```python
from build123d import *

# Parameters (mm, degrees)
F0_R      = 2
F0_R_2    = 1.25
F1_DEPTH  = 2.5
F2_DEPTH  = 8.5
F3_R      = 1.25
F2_FACE_R = 1.25
F4_DEPTH  = 1.5
F5_R      = 0.25


with BuildPart() as f1:
    # F0 (on Top) → F1 (new body)
    with BuildSketch(Plane.XY):
        Circle(F0_R)
        Circle(F0_R_2, mode=Mode.SUBTRACT)
    extrude(amount=F1_DEPTH)

    # F0 (on Top) → F2 (join)
    with BuildSketch(Plane.XY):
        Circle(F0_R_2)
    extrude(amount=F2_DEPTH)

    # F0 (on Top) + F3 (on face) + F2_face (on face) → F4 (cut)
    with BuildSketch(Plane.XY):
        Circle(F0_R_2)
    with BuildSketch(Plane.XY):
        Polygon((-0.8660254038, -1.5), (0.8660254038, -1.5), (1.7320508076, 0), (0.8660254038, 1.5), (-0.8660254038, 1.5), (-1.7320508076, 0), align=None)
        Circle(F3_R, mode=Mode.SUBTRACT)
        Circle(F3_R)
    with BuildSketch(Plane.XY.offset(8.5)):
        Circle(F2_FACE_R)
    extrude(amount=F4_DEPTH, mode=Mode.SUBTRACT)

    # F5
    f5_edges = [f1.edges().sort_by_distance(p)[0] for p in [
        (-1.25, 0, 2.5),
        (-2, 0, 2.5),
        (-2, 0, 0),
    ]]
    fillet(f5_edges, radius=F5_R)


solid = f1.part
```
Verification items for the finished model (mm, model axes). A direction names the side the tool comes from. Round coordinates to 2 decimals unless told otherwise and drop trailing zeros. Write each loop counter-clockwise with the first axis right and the second up, starting at its lowest first coordinate (ties: lowest second). Pieces come first, ordered by that corner, then holes.
1. Gauge pin test, flat ends, axial feed: P1, Ø2, axis at x = -1, z = 5, coming from the -Y side; P2, Ø1.5, axis at x = -0.5, y = 0.5, coming from the -Z side. Record the tip position at first contact, or that the pin passes through.
2. Scan lines: L1, parallel to X at y = -0.9, z = 1; L2, parallel to Z at x = 1.45, y = -0.9; L3, parallel to Z at x = 0.15, y = 0.95. Record each from-to range of solid material in increasing order.
3. Access from +Z, -Z, +X, -X, +Y, -Y to the whole of each face (thin tool, end or side, straight path). Record for faces 4 (the flat face through (0, -1.5, 1)), 5 (the cylindrical face through (0, -2, 1)).
4. Draft check along X on faces 1 (the flat face through (-1.305, -0.74, 0.74)), 2 (the cylindrical face through (-0.27, -1.22, 5.58)), 3 (the flat face through (0, 0, 8.5)). Enter one of: +X half, -X half, draft (parallel to the pull), parting line (faces both ways), or undercut.
5. Section check A-A on x = 0. Enter the section's corners in (y, z), plus the area to 3 significant figures.
6. Section check B-B on z = 4. Enter the section's corners in (x, y), plus the area to 3 significant figures.
Answer:
1. P1: stops at y = -1.25
1. P2: stops at z = 1.5
2. L1: x = -1.79 to -1.21, 1.21 to 1.79
2. L2: z = 0 to 2.5
2. L3: z = 1.5 to 8.5
3. face 4: -Z
3. face 5: +Z, -Z
4. face 1: undercut
4. face 2: parting line
4. face 3: draft
5. outline: (-2, 0.25) arc R0.25 ccw to (-1.75, 0) - (-1.5, 0) - (-1.5, 1.5) - (1.5, 1.5) - (1.5, 0) - (1.75, 0) arc R0.25 ccw to (2, 0.25) - (2, 2.25) arc R0.25 ccw to (1.75, 2.5) - (1.5, 2.5) arc R0.25 cw to (1.25, 2.75) - (1.25, 8.5) - (-1.25, 8.5) - (-1.25, 2.75) arc R0.25 cw to (-1.5, 2.5) - (-1.75, 2.5) arc R0.25 ccw to (-2, 2.25) - close
5. area: 20.5 mm2
6. outline: circle Ø2.5 at (0, 0)
6. area: 4.91 mm2
